Geometry: final body of the model. Coordinates: model frame, mm. Face numbers are marked on the shaded views. A direction names the side the tool comes from. Round coordinates to 2 decimals unless told otherwise and drop trailing zeros. Order: outer loops, then holes, each group sorted by start corner. A loop starts at its lowest first (then second) coordinate and runs counter-clockwise, first axis right, second up. Notation, with made-up numbers: M -26,69.25 L -10,69.25 A17 ccw -10,99.25 Z; hole C 86.25,39.5 d9. An arc over 180 degrees is marked long. Put each result on its own line as item: value. Start each with the question number.
1) Section D-D, the plane z = 18.5. Return loops of the section in (x, y), then the cut area to 3 significant figures.
2) Section B-B, the plane z = 6.5. Return loops of the section in (x, y).
3) Section C-C, the plane y = 28. Return loops of the section in (x, z) (3 decimals).
4) Access query for the marked faces 4, 5 and 6. Directions: +Z, -Z, +X, -X, +Y, -Y. A direction counts if a zero-diameter tool reaches every point of the face in a straight line with its end or side. Return the directions, or none.
5) Draft query along X for the marked faces 1, 2 and 3. Return one class per face: pulls with the +X half, pulls with the -X half, needs draft (parallel to the pull), parting line crosses it, or undercut.
6) Section A-A, the plane x = 25. Return loops of the section in (y, z) (3 decimals), then the cut area to 3 significant figures.
7) First-contact query: P1, Ø5.5, axis at y = -34, z = -7, coming from the -X side; P2, Ø12, axis at x = 26.5, z = 7, coming from the -Y side; P3, Ø2.5, axis at y = -8, z = -6.5, coming from the -X side (3 decimals); P4, Ø2, axis at x = -9, y = 59, coming from the -Z side (3 decimals). Flat tips, straight axial feed; report the tip coordinate or a pass-through.
8) Material intervals for probe 1 along Y at (x, z) = (-20.5, 6); probe 2 along X at (y, z) = (60.5, 9); probe 3 along Y at (x, z) = (-7, -0.5), sorted ascending. Write a range as [from, to].
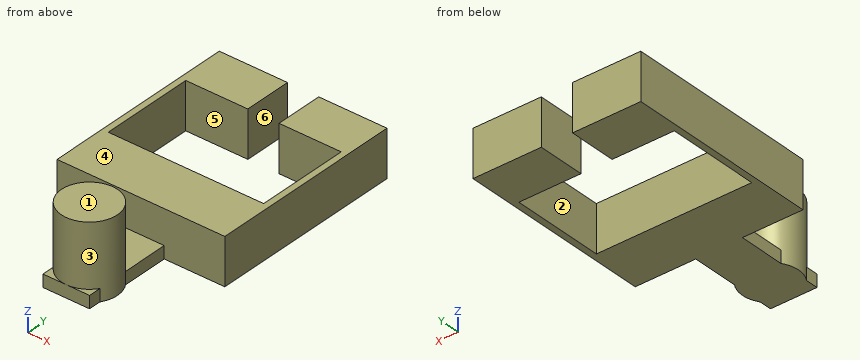
from build123d import *

# Parameters (mm, degrees)
SKETCH1_W            = 68.64096
SKETCH1_H            = 79.975020836
MAIN_BODY_DEPTH      = 9.525
SKETCH2_W            = 63.56096
SKETCH2_H            = 38.227
LOWER_T_CAVITY_DEPTH = 90.088729956
SKETCH3_W            = 12.7508
SKETCH3_H            = 19.558
TOP_SLOT_DEPTH       = 90.088729956
SKETCH4_W            = 19.05
SKETCH4_H            = 36.82365
HANGER_DEPTH         = 5.08
SKETCH5_R            = 11.42365
STRAP_PIN_DEPTH      = 30.48


with BuildPart() as part:
    # Sketch1 → Main-Body (new, symmetric)
    with BuildSketch(Plane.XY):
        with Locations((0, 39.987510418)):
            Rectangle(SKETCH1_W, SKETCH1_H)
    extrude(amount=MAIN_BODY_DEPTH, both=True)

    # Sketch2 → Lower-T-Cavity (cut, through all)
    with BuildSketch(Plane.XY.offset(9.525)):
        with Locations((0, 41.303520836)):
            Rectangle(SKETCH2_W, SKETCH2_H)
    extrude(amount=-LOWER_T_CAVITY_DEPTH, mode=Mode.SUBTRACT)

    # Sketch3 → Top-Slot (cut, through all)
    with BuildSketch(Plane.XY.offset(9.525)):
        with Locations((0, 70.196020836)):
            Rectangle(SKETCH3_W, SKETCH3_H)
    extrude(amount=-TOP_SLOT_DEPTH, mode=Mode.SUBTRACT)

    # Sketch4 → Hanger (add)
    with BuildSketch(Plane(origin=(0, 0, -9.525), x_dir=(-1, 0, 0), z_dir=(0, 0, -1))):
        with Locations((0, -18.411825)):
            Rectangle(SKETCH4_W, SKETCH4_H)
    extrude(amount=-HANGER_DEPTH)

    # Sketch5 → Strap-Pin (add)
    with BuildSketch(Plane(origin=(0, 0, -9.525), x_dir=(-1, 0, 0), z_dir=(0, 0, -1))):
        with Locations((0, -25.4)):
            Circle(SKETCH5_R)
    extrude(amount=-STRAP_PIN_DEPTH)


solid = part.part
Result sheet:
1. outline: C 0,-25.4 d22.85
1. area: 410 mm2
2. outline: M -34.32,0 L 34.32,0 L 34.32,79.98 L 6.38,79.98 L 6.38,60.42 L 31.78,60.42 L 31.78,22.19 L -31.78,22.19 L -31.78,60.42 L -6.38,60.42 L -6.38,79.98 L -34.32,79.98 Z; C 0,-25.4 d22.85
3. outline: M -34.32,-9.525 L -31.78,-9.525 L -31.78,9.525 L -34.32,9.525 Z; M 31.78,-9.525 L 34.32,-9.525 L 34.32,9.525 L 31.78,9.525 Z
4. face 4: +Z, +X, -X, +Y
4. face 5: +Z, -Z
4. face 6: +Z, -Z, +Y
5. face 1: needs draft
5. face 2: undercut
5. face 3: parting line crosses it
6. outline: M 0,-9.525 L 22.19,-9.525 L 22.19,9.525 L 0,9.525 Z; M 60.417,-9.525 L 79.975,-9.525 L 79.975,9.525 L 60.417,9.525 Z
6. area: 795 mm2
7. P1: stops at x = -9.81
7. P2: stops at y = 0
7. P3: stops at x = -9.525
7. P4: passes through
8. probe 1: y = [0, 22.19], [60.42, 79.98]
8. probe 2: x = [-34.32, -6.38], [6.38, 34.32]
8. probe 3: y = [-34.43, -16.37], [0, 22.19], [60.42, 79.98]
